Here's how the part is built. I have some questions about the finished solid (model axes, mm). A direction names the side the tool comes from. Round coordinates to 2 decimals unless told otherwise and drop trailing zeros. Order: outer loops, then holes, each group sorted by start corner. A loop starts at its lowest first (then second) coordinate and runs counter-clockwise, first axis right, second up. Notation, with made-up numbers: (-37.75, 58) - (-0.75, 58) arc R20 ccw to (-0.75, 62) - close; hole circle Ø7 at (84, 15). An arc over 180 degrees is marked (long way). Answer as a JSON object with one key per item and string values.
Autodesk Inventor part; units mm, degrees
ref_plane "YZ Plane" through (0, 0, 0) normal (1, 0, 0) x (0, 1, 0)
ref_plane "XZ Plane" through (0, 0, 0) normal (0, 1, 0) x (-1, 0, 0)
ref_plane "XY Plane" through (0, 0, 0) normal (0, 0, 1) x (1, 0, 0)
sketch "Sketch1" plane through (0, 0, 0) normal (0, 1, 0) x (-1, 0, 0)
  line L0 (-25, -25) -> (25, -25)
  line L1 (25, -25) -> (25, 25)
  line L2 (25, 25) -> (-25, 25)
  line L3 (-25, 25) -> (-25, -25)
  line L4 (-25, -25) -> (25, 25) construction
  line L5 (25, -25) -> (-25, 25) construction
  point P0 (0, 0)
  dimension "d7" = 50
  dimension "d8" = 50
extrude "Base plate" add sketch "Sketch1" along normal blind 3
sketch "Sketch2" plane through (0, 3, 0) normal (0, 1, 0) x (1, 0, 0)
  circle A0 centre (10, -13) radius 6.75
  line L0 (-25, 25) -> (-25, -25)
  line L1 (-25, -25) -> (25, -25)
  point P0 (0, 0)
  dimension "d2" = 13.5
  dimension "d3" = 35
  dimension "d4" = 12
extrude "Tuimel" cut sketch "Sketch2" against normal through all
sketch "Sketch3" plane through (0, 3, 0) normal (0, 1, 0) x (1, 0, 0)
  circle A0 centre (-15, -13) radius 6.25
  line L0 (-25, 25) -> (-25, -25)
  line L1 (-25, -25) -> (25, -25)
  point P0 (0, 0)
  point P1 (5.9214, -25)
  point P2 (-5.9214, -25)
  dimension "d9" = 12.5
  dimension "d10" = 10
  dimension "d11" = 12
extrude "Button" cut sketch "Sketch3" against normal through all
sketch "Sketch5" plane through (0, 3, 0) normal (0, 1, 0) x (1, 0, 0)
  circle A0 centre (-10, 10) radius 9.5
  line L0 (-25, 25) -> (-25, -25)
  line L1 (-25, -25) -> (25, -25)
  point P0 (0, 0)
  dimension "d19" = 19
  dimension "d20" = 15
  dimension "d21" = 35
extrude "Sleutel 19" cut sketch "Sketch5" against normal through all
sketch "Sketch6" plane through (0, 3, 0) normal (0, 1, 0) x (1, 0, 0)
  line L0 (6, 0) -> (20, 0)
  line L1 (20, 0) -> (20, 20)
  line L2 (20, 20) -> (6, 20)
  line L3 (6, 20) -> (6, 0)
  line L4 (6, 0) -> (20, 20) construction
  line L5 (20, 0) -> (6, 20) construction
  line L6 (25, 25) -> (-25, 25)
  line L7 (25, -25) -> (25, 25)
  point P0 (0, 0)
  point P1 (13, 10)
  dimension "d24" = 14
  dimension "d25" = 20
  dimension "d26" = 5
  dimension "d27" = 5
extrude "Schakelaar" cut sketch "Sketch6" against normal through all
properties part number "Holes_Test"
1. Imagine slicing it at B-B (x = 10). List the corners of the cut face in (y, z) for me, plus the area to 3 significant figures.
Responses:
{"outline": "(0, -25) - (3, -25) - (3, -20) - (0, -20) - close; (0, 0) - (3, 0) - (3, 6.25) - (0, 6.25) - close; (0, 19.75) - (3, 19.75) - (3, 25) - (0, 25) - close", "area": "49.5 mm2"}
2. Imagine slicing it at A-A (z = -10). List the corners of the cut face in (x, y) for me.
Responses:
{"outline": "(-25, 0) - (-19.5, 0) - (-19.5, 3) - (-25, 3) - close; (-0.5, 0) - (6, 0) - (6, 3) - (-0.5, 3) - close; (20, 0) - (25, 0) - (25, 3) - (20, 3) - close"}
3. Thinking about a two-plate mould opening in X: for faces 3 (the face through (25, 1, 0)), 4 (the face through (-25, 1, 0)), 5 (the face through (13, 2, -20)), which applies, pulls with the +X half, pulls with the -X half, needs draft (parallel to the pull), parting line crosses it, or undercut?
Responses:
{"face 3": "pulls with the +X half", "face 4": "pulls with the -X half", "face 5": "undercut"}
4. If I drill on L1, parallel to X at y = 0.7, z = -10; L2, parallel to X at y = 2.2, z = 13; L3, parallel to Z at x = 18.5, y = 1.45, over which ranges is the centre line in solid material (lowest first)? Write a range as [from, to].
Responses:
{"L1": "[-25, -19.5], [-0.5, 6], [20, 25]", "L2": "[-25, -21.25], [-8.75, 3.25], [16.75, 25]", "L3": "[-25, -20], [0, 25]"}
5. For faces 1 (the face through (0, 0, 0)), 2 (the face through (6, 2, -10)), which set-ups out of +Z, -Z, +X, -X, +Y, -Y let a thin tool reach every point of the face, with its end or its side?
Responses:
{"face 1": "+Z, -Z, +X, -X, -Y", "face 2": "+Y, -Y"}
6. Imagine slicing it at C-C (y = 0.95). List the corners of the cut face in (x, z) for me, plus the area to 3 significant figures.
Responses:
{"outline": "(-25, -25) - (25, -25) - (25, 25) - (-25, 25) - close; hole circle Ø12.5 at (-15, 13); hole circle Ø19 at (-10, -10); hole circle Ø13.5 at (10, 13); hole (6, -20) - (20, -20) - (20, 0) - (6, 0) - close", "area": "1,670 mm2"}
7. Imagine slicing it at D-D (x = 19). List the corners of the cut face in (y, z) for me.
Responses:
{"outline": "(0, -25) - (3, -25) - (3, -20) - (0, -20) - close; (0, 0) - (3, 0) - (3, 25) - (0, 25) - close"}
